```python
from build123d import *

# Parameters (mm, degrees)
F0_W     = 24
F0_H     = 2
F1_DEPTH = 4
F2_SIZE2 = 2
F2_SIZE  = 0.5
F3_R     = 2


with BuildPart() as f1:
    # F0 (on Top) → F1 (new body)
    with BuildSketch(Plane.XY):
        Polygon((-12, 13), (-14, 13), (-14, -13), (-12, -13), (-12, -11), (-12, 11), align=None)
        with Locations((0, 12)):
            Rectangle(F0_W, F0_H)
        Polygon((14, 13), (12, 13), (12, 11), (12, -11), (12, -13), (14, -13), align=None)
        with Locations((0, -12)):
            Rectangle(F0_W, F0_H)
    extrude(amount=F1_DEPTH)

    # F2
    f2_edges = [f1.edges().sort_by_distance(p)[0] for p in [
        (-12, 0, 4),
        (0, 11, 4),
        (12, 0, 4),
        (0, -11, 4),
    ]]
    f2_side = f1.faces().sort_by_distance((-13.617901, 0, 4))[0]
    chamfer(f2_edges, length=F2_SIZE, length2=F2_SIZE2, reference=f2_side)

    # F3
    f3_edges = [f1.edges().sort_by_distance(p)[0] for p in [
        (14, -13, 2),
        (-14, -13, 2),
        (-14, 13, 2),
        (14, 13, 2),
    ]]
    fillet(f3_edges, radius=F3_R)


solid = f1.part
```
Here's how the part is built. I have some questions about the finished solid (model axes, mm). A direction names the side the tool comes from. Give positions to 0.01 mm unless a question says otherwise; leave off trailing zeros. Write each loop counter-clockwise with the first axis right and the second up, starting at its lowest first coordinate (ties: lowest second). Pieces come first, ordered by that corner, then holes.
(1) Imagine slicing it at C-C, the plane x = 1. Write out the boundary of the cut face in (y, z), and give its area (3 significant figures).
Output values:
outline: (-13, 0) - (-11, 0) - (-11, 2) - (-11.5, 4) - (-13, 4) - close; (11, 0) - (13, 0) - (13, 4) - (11.5, 4) - (11, 2) - close
area: 15.0 mm2
(2) On a 3-axis mill with a long thin cutter (end or side, diameter ignored), from which of +Z, -Z, +X, -X, +Y, -Y can I reach the whole of each face in a straight line? I mean faces 1 (the face through (0, -11, 1)), 2 (the face through (0, -13, 2)), 3 (the face through (12.246, 0.161, 2.986)). Say none if no direction works.
Output values:
face 1: +Z, -Z
face 2: +Z, -Z, +X, -X, -Y
face 3: +Z
(3) Thinking about a two-plate mould opening in X: for faces 4 (the face through (0, 13, 2)), 5 (the face through (13.43, 12.4, 2.03)), 6 (the face through (-14, 0, 2)), 7 (the face through (-12, 0, 1)), which applies, pulls with the +X half, pulls with the -X half, needs draft (parallel to the pull), parting line crosses it, or undercut?
Output values:
face 4: needs draft
face 5: pulls with the +X half
face 6: pulls with the -X half
face 7: undercut
(4) If I drill on L1, parallel to Y at x = 3, z = 0.3; L2, parallel to X at y = -7.75, z = 1.7; L3, parallel to Y at x = 0, z = 3.35, over which ranges is the centre line in solid material (lowest first)?
Output values:
L1: y = -13 to -11, 11 to 13
L2: x = -14 to -12, 12 to 14
L3: y = -13 to -11.34, 11.34 to 13
(5) Imagine slicing it at B-B, the plane y = 7.25. Write out the boundary of the cut face in (x, z), and give its area (3 significant figures).
Output values:
outline: (-14, 0) - (-12, 0) - (-12, 2) - (-12.5, 4) - (-14, 4) - close; (12, 0) - (14, 0) - (14, 4) - (12.5, 4) - (12, 2) - close
area: 15.0 mm2
(6) Will this pin go through, and if not, where does the flat tip stop? pin 1 (1 mm diameter, centred on x = -6, y = 10, fed in from -Z).
Output values:
pin 1: passes through
(7) Imagine slicing it at A-A, the plane z = 2.8. Write out the boundary of the cut face in (x, y), and give its area (3 significant figures).
Output values:
outline: (-14, -11) arc R2 ccw to (-12, -13) - (12, -13) arc R2 ccw to (14, -11) - (14, 11) arc R2 ccw to (12, 13) - (-12, 13) arc R2 ccw to (-14, 11) - close; hole (-12.2, -11.2) - (12.2, -11.2) - (12.2, 11.2) - (-12.2, 11.2) - close
area: 178 mm2
(8) Imagine slicing it at D-D, the plane z = 1.15. Write out the boundary of the cut face in (x, y).
Output values:
outline: (-14, -11) arc R2 ccw to (-12, -13) - (12, -13) arc R2 ccw to (14, -11) - (14, 11) arc R2 ccw to (12, 13) - (-12, 13) arc R2 ccw to (-14, 11) - close; hole (-12, -11) - (12, -11) - (12, 11) - (-12, 11) - close
